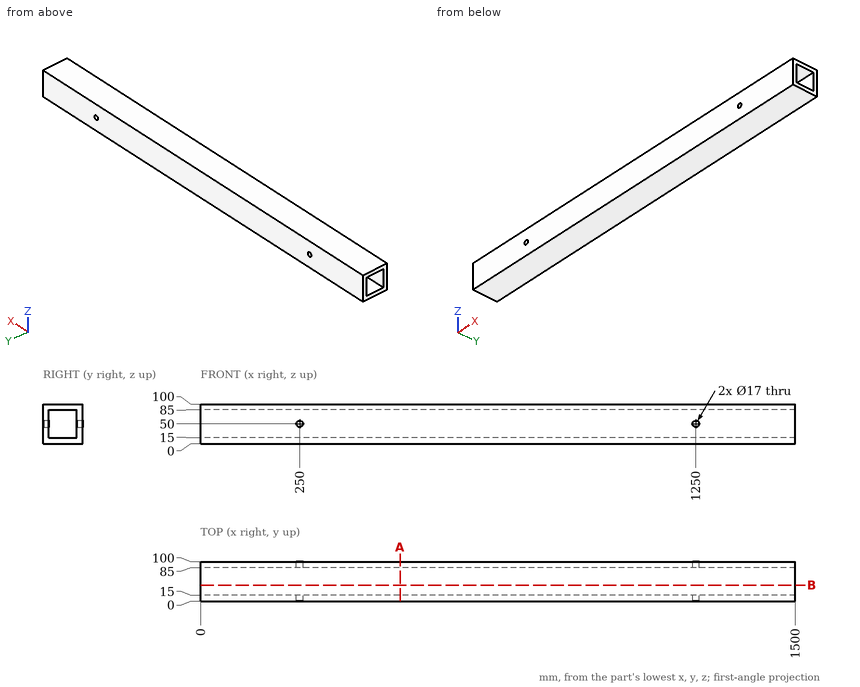
Geometry check sheet. Reference: drawing and pictorial views, mm from the part's lowest x, y, z. Round coordinates to 2 decimals unless told otherwise and drop trailing zeros. Loops run counter-clockwise (first coordinate to the right, second up) from the corner with the lowest first, then second, coordinate; pieces in that order, holes last. Notation, with made-up numbers: (62, 43.25) - (104, 43.25) arc R15 cw to (104, 71.25) - close; hole circle Ø3 at (22.5, -34). An arc over 180 degrees is marked (long way). One line per question, with ' | ' between items. Start each with the question number.
1. Cross-section at B-B on y = 40.5. Record the cut outline in (x, z).
2. Scan lines: line 1 (Y direction, x = 1033, z = 27); line 2 (Z direction, x = 250, y = 94.25). Record each from-to range of solid material in increasing order. Write a range as [from, to].
3. Cross-section at A-A on x = 503.5. Record the cut outline in (y, z).
Taken from the geometry:
1) outline: (0, 0) - (1500, 0) - (1500, 15) - (0, 15) - close; (0, 85) - (1500, 85) - (1500, 100) - (0, 100) - close
2) line 1: [0, 15], [85, 100] | line 2: [0, 41.5], [58.5, 100]
3) outline: (0, 0) - (100, 0) - (100, 100) - (0, 100) - close; hole (15, 15) - (85, 15) - (85, 85) - (15, 85) - close
